Geometry: final body of the model. Coordinates: model frame, mm. A direction names the side the tool comes from. Give positions to 0.01 mm unless a question says otherwise; leave off trailing zeros. Loops run counter-clockwise (first coordinate to the right, second up) from the corner with the lowest first, then second, coordinate; pieces in that order, holes last.
1. Draft query along Z for faces 1 (the face through (88.35, 3, -10)), 2 (the face through (79, 0, -132)), 3 (the face through (79, 3, -260)). Return one class per face: +Z half, -Z half, draft (parallel to the pull), parting line (faces both ways), or undercut.
2. Section C-C, the plane z = -67. Output: boundary loops of the cut face in (x, y), then the cut area to 3 significant figures.
3. Material intervals for line 1 along X through (y, z) = (5.25, -223); line 2 along Z through (x, y) = (70, 5); line 3 along X through (y, z) = (4.75, -45), sorted ascending.
4. Access query for faces 4 (the face through (160, 3, -128)), 5 (the face through (151.65, 3, -10)). Directions: +Z, -Z, +X, -X, +Y, -Y. A direction counts if a zero-diameter tool reaches every point of the face in a straight line with its end or side. Return the directions, or none.
5. Section D-D, the plane y = 4.75. State how many separate pieces and enclosed holes the cut face has, then the cut area to 3 significant figures.
6. First-contact query: P1, Ø2.5, axis at x = 50, z = -250, coming from the +Y side; P2, Ø3, axis at y = 2.5, z = -11, coming from the -X side. Flat tips, straight axial feed; report the tip coordinate or a pass-through.
7. Section B-B, the plane x = 81. Output: boundary loops of the cut face in (y, z), then the cut area to 3 significant figures.
8. Section A-A, the plane z = -170. Output: boundary loops of the cut face in (x, y), then the cut area to 4 significant figures.
from build123d import *

# Parameters (mm, degrees)
SKETCH1_W           = 160
SKETCH1_H           = 260
SKETCH1_R           = 25
SKETCH1_R_2         = 2.25
SKETCH1_R_3         = 1.175
SKETCH1_R_4         = 1.65
BOSS_EXTRUDE1_DEPTH = 6.35
SKETCH2_R           = 1.7
CUT_EXTRUDE1_DEPTH  = 306.352783678


with BuildPart() as part:
    # Sketch1 → Boss-Extrude1 (new body)
    with BuildSketch(Plane(origin=(0, 0, 0), x_dir=(1, 0, 0), z_dir=(0, 1, 0))):
        with Locations((80, 130)):
            Rectangle(SKETCH1_W, SKETCH1_H)
        with Locations(Location((87.5, 170, 0), (0, 0, 270))):
            Circle(SKETCH1_R, mode=Mode.SUBTRACT)
        with Locations(Location((87.5, 45, 0), (0, 0, 270))):
            Circle(SKETCH1_R, mode=Mode.SUBTRACT)
        with Locations(Location((118.125, 116.955944018, 0), (0, 0, 270))):
            Circle(SKETCH1_R_2, mode=Mode.SUBTRACT)
        with Locations(Location((56.875, 116.955944018, 0), (0, 0, 270))):
            Circle(SKETCH1_R_2, mode=Mode.SUBTRACT)
        with Locations(Location((56.875, 223.044055982, 0), (0, 0, 270))):
            Circle(SKETCH1_R_2, mode=Mode.SUBTRACT)
        with Locations(Location((118.125, 223.044055982, 0), (0, 0, 270))):
            Circle(SKETCH1_R_2, mode=Mode.SUBTRACT)
        with Locations(Location((5.475532842, 135.298909731, 0), (0, 0, 270))):
            Circle(SKETCH1_R_3, mode=Mode.SUBTRACT)
        with Locations(Location((9.516263037, 126.701090269, 0), (0, 0, 270))):
            Circle(SKETCH1_R_3, mode=Mode.SUBTRACT)
        with Locations(Location((10, 250, 0), (0, 0, 270))):
            Circle(SKETCH1_R_4, mode=Mode.SUBTRACT)
        with Locations(Location((30, 250, 0), (0, 0, 270))):
            Circle(SKETCH1_R_4, mode=Mode.SUBTRACT)
        with Locations(Location((50, 250, 0), (0, 0, 270))):
            Circle(SKETCH1_R_4, mode=Mode.SUBTRACT)
        with Locations(Location((70, 250, 0), (0, 0, 270))):
            Circle(SKETCH1_R_4, mode=Mode.SUBTRACT)
        with Locations(Location((90, 250, 0), (0, 0, 270))):
            Circle(SKETCH1_R_4, mode=Mode.SUBTRACT)
        with Locations(Location((110, 250, 0), (0, 0, 270))):
            Circle(SKETCH1_R_4, mode=Mode.SUBTRACT)
        with Locations(Location((130, 250, 0), (0, 0, 270))):
            Circle(SKETCH1_R_4, mode=Mode.SUBTRACT)
        with Locations(Location((150, 250, 0), (0, 0, 270))):
            Circle(SKETCH1_R_4, mode=Mode.SUBTRACT)
        with BuildLine():
            Line((8.35, 6.5), (8.35, 13.5))
            ThreePointArc((8.35, 13.5), (10, 15.15), (11.65, 13.5))
            Line((11.65, 13.5), (11.65, 6.5))
            ThreePointArc((11.65, 6.5), (10, 4.85), (8.35, 6.5))
        make_face(mode=Mode.SUBTRACT)
        with BuildLine():
            Line((31.65, 6.5), (31.65, 13.5))
            ThreePointArc((31.65, 13.5), (30, 15.15), (28.35, 13.5))
            Line((28.35, 13.5), (28.35, 6.5))
            ThreePointArc((28.35, 6.5), (30, 4.85), (31.65, 6.5))
        make_face(mode=Mode.SUBTRACT)
        with BuildLine():
            Line((51.65, 6.5), (51.65, 13.5))
            ThreePointArc((51.65, 13.5), (50, 15.15), (48.35, 13.5))
            Line((48.35, 13.5), (48.35, 6.5))
            ThreePointArc((48.35, 6.5), (50, 4.85), (51.65, 6.5))
        make_face(mode=Mode.SUBTRACT)
        with BuildLine():
            Line((71.65, 6.5), (71.65, 13.5))
            ThreePointArc((71.65, 13.5), (70, 15.15), (68.35, 13.5))
            Line((68.35, 13.5), (68.35, 6.5))
            ThreePointArc((68.35, 6.5), (70, 4.85), (71.65, 6.5))
        make_face(mode=Mode.SUBTRACT)
        with BuildLine():
            Line((91.65, 6.5), (91.65, 13.5))
            ThreePointArc((91.65, 13.5), (90, 15.15), (88.35, 13.5))
            Line((88.35, 13.5), (88.35, 6.5))
            ThreePointArc((88.35, 6.5), (90, 4.85), (91.65, 6.5))
        make_face(mode=Mode.SUBTRACT)
        with BuildLine():
            Line((111.65, 6.5), (111.65, 13.5))
            ThreePointArc((111.65, 13.5), (110, 15.15), (108.35, 13.5))
            Line((108.35, 13.5), (108.35, 6.5))
            ThreePointArc((108.35, 6.5), (110, 4.85), (111.65, 6.5))
        make_face(mode=Mode.SUBTRACT)
        with BuildLine():
            Line((131.65, 6.5), (131.65, 13.5))
            ThreePointArc((131.65, 13.5), (130, 15.15), (128.35, 13.5))
            Line((128.35, 13.5), (128.35, 6.5))
            ThreePointArc((128.35, 6.5), (130, 4.85), (131.65, 6.5))
        make_face(mode=Mode.SUBTRACT)
        with BuildLine():
            Line((151.65, 6.5), (151.65, 13.5))
            ThreePointArc((151.65, 13.5), (150, 15.15), (148.35, 13.5))
            Line((148.35, 13.5), (148.35, 6.5))
            ThreePointArc((148.35, 6.5), (150, 4.85), (151.65, 6.5))
        make_face(mode=Mode.SUBTRACT)
    extrude(amount=BOSS_EXTRUDE1_DEPTH)

    # Sketch2 → Cut-Extrude1 (cut, through all)
    with BuildSketch(Plane(origin=(0, 6.35, 0), x_dir=(1, 0, 0), z_dir=(0, 1, 0))):
        with Locations(Location((27.663890721, 60.64097268, 0), (0, 0, 270))):
            Circle(SKETCH2_R)
        with Locations(Location((42.063890721, 86.95902732, 0), (0, 0, 270))):
            Circle(SKETCH2_R)
    extrude(amount=-CUT_EXTRUDE1_DEPTH, mode=Mode.SUBTRACT)


solid = part.part
Answers below:
1. face 1: undercut
1. face 2: draft
1. face 3: -Z half
2. outline: (0, 0) - (75.63, 0) - (75.63, 6.35) - (0, 6.35) - close; (99.37, 0) - (160, 0) - (160, 6.35) - (99.37, 6.35) - close
2. area: 865 mm2
3. line 1: x = 0 to 54.63, 59.12 to 115.88, 120.37 to 160
3. line 2: z = -260 to -251.65, -248.35 to -187.85, -152.15 to -62.85, -27.15 to -15.15, -4.85 to 0
3. line 3: x = 0 to 62.5, 112.5 to 160
4. face 4: +Z, -Z, +X, +Y, -Y
4. face 5: +Y, -Y
5. separate pieces: 1
5. enclosed holes: 26
5. area: 37,300 mm2
6. P1: passes through
6. P2: stops at x = 0
7. outline: (0, -260) - (6.35, -260) - (6.35, -194.14) - (0, -194.14) - close; (0, -145.86) - (6.35, -145.86) - (6.35, -69.14) - (0, -69.14) - close; (0, -20.86) - (6.35, -20.86) - (6.35, 0) - (0, 0) - close
7. area: 1,040 mm2
8. outline: (0, 0) - (62.5, 0) - (62.5, 6.35) - (0, 6.35) - close; (112.5, 0) - (160, 0) - (160, 6.35) - (112.5, 6.35) - close
8. area: 698.5 mm2
